from build123d import *

# Parameters (mm, degrees)
SKETCH1_R           = 36
SKETCH1_R_2         = 31.1
BOSS_EXTRUDE1_DEPTH = 15
SKETCH2_R           = 36
BOSS_EXTRUDE2_DEPTH = 5
SKETCH3_R           = 22.5
CUT_EXTRUDE1_DEPTH  = 5
SKETCH4_R           = 5
BOSS_EXTRUDE3_DEPTH = 20
SKETCH7_R           = 2.25
CUT_EXTRUDE2_DEPTH  = 21


with BuildPart() as part:
    # Sketch1 → Boss-Extrude1 (new body)
    with BuildSketch(Plane.XY):
        Circle(SKETCH1_R)
        Circle(SKETCH1_R_2, mode=Mode.SUBTRACT)
    extrude(amount=BOSS_EXTRUDE1_DEPTH)

    # Sketch2 → Boss-Extrude2 (add)
    with BuildSketch(Plane.XY.offset(15)):
        Circle(SKETCH2_R)
    extrude(amount=BOSS_EXTRUDE2_DEPTH)

    # Sketch3 → Cut-Extrude1 (cut)
    with BuildSketch(Plane.XY.offset(20)):
        Circle(SKETCH3_R)
    extrude(amount=-CUT_EXTRUDE1_DEPTH, mode=Mode.SUBTRACT)

    # Sketch4 → Boss-Extrude3 (add)
    with BuildSketch(Plane(origin=(0, 0, 0), x_dir=(-1, 0, 0), z_dir=(0, 0, -1))):
        with Locations((0, 36.1)):
            Circle(SKETCH4_R)
        with Locations((31.263517077, 18.05)):
            Circle(SKETCH4_R)
        with Locations((31.263517077, -18.05)):
            Circle(SKETCH4_R)
        with Locations((0, -36.1)):
            Circle(SKETCH4_R)
        with Locations((-31.263517077, -18.05)):
            Circle(SKETCH4_R)
        with Locations((-31.263517077, 18.05)):
            Circle(SKETCH4_R)
    extrude(amount=-BOSS_EXTRUDE3_DEPTH)

    # Sketch7 → Cut-Extrude2 (cut, through all)
    with BuildSketch(Plane(origin=(0, 0, 0), x_dir=(-1, 0, 0), z_dir=(0, 0, -1))):
        with Locations((-31.263517077, 18.05)):
            Circle(SKETCH7_R)
        with Locations((0, 36.1)):
            Circle(SKETCH7_R)
        with Locations((31.263517077, 18.05)):
            Circle(SKETCH7_R)
        with Locations((31.263517077, -18.05)):
            Circle(SKETCH7_R)
        with Locations((0, -36.1)):
            Circle(SKETCH7_R)
        with Locations((-31.263517077, -18.05)):
            Circle(SKETCH7_R)
    extrude(amount=-CUT_EXTRUDE2_DEPTH, mode=Mode.SUBTRACT)


solid = part.part
Input: part model. Units: mm. Frame: model coordinates. A direction names the side the tool comes from. Give positions to 0.01 mm unless a question says otherwise; leave off trailing zeros. Loops run counter-clockwise (first coordinate to the right, second up) from the corner with the lowest first, then second, coordinate; pieces in that order, holes last. Notation, with made-up numbers: M -12.5,61.5 L 34.5,61.5 A21 ccw 34.5,79.5 Z; hole C 11,-15.5 d9. An arc over 180 degrees is marked long. Use one line per item in the form item = value.
1. Section query A-A, the plane y = 0. Return the cut outline in (x, z), and give its area (3 significant figures).
Numbers:
outline = M -36,0 L -31.1,0 L -31.1,15 L -22.5,15 L -22.5,20 L -36,20 Z; M 22.5,15 L 31.1,15 L 31.1,0 L 36,0 L 36,20 L 22.5,20 Z
area = 282 mm²
2. Section query B-B, the plane z = 9.25. Return the cut outline in (x, y), and give its area (3 significant figures).
Numbers:
outline = M -33.37,-13.51 A5 ccw long -28.39,-22.14 A36 ccw -4.98,-35.65 A5 ccw long 4.98,-35.65 A36 ccw 28.39,-22.14 A5 ccw long 33.37,-13.51 A36 ccw 33.37,13.51 A5 ccw long 28.39,22.14 A36 ccw 4.98,35.65 A5 ccw long -4.98,35.65 A36 ccw -28.39,22.14 A5 ccw long -33.37,13.51 A36 ccw Z; hole C -31.26,-18.05 d4.5; hole C -31.26,18.05 d4.5; hole C 0,0 d62.2; hole C 0,-36.1 d4.5; hole C 0,36.1 d4.5; hole C 31.26,-18.05 d4.5; hole C 31.26,18.05 d4.5
area = 1,190 mm²
3. Section query D-D, the plane y = 18.05. Return the cut outline in (x, z).
Numbers:
outline = M -36.26,0 L -33.51,0 L -33.51,20 L -36.26,20 Z; M -29.01,0 L -25.33,0 L -25.33,15 L -13.43,15 L -13.43,20 L -29.01,20 Z; M 13.43,15 L 25.33,15 L 25.33,0 L 29.01,0 L 29.01,20 L 13.43,20 Z; M 33.51,0 L 36.26,0 L 36.26,20 L 33.51,20 Z
4. Section query C-C, the plane x = 0. Return the cut outline in (y, z).
Numbers:
outline = M -41.1,0 L -38.35,0 L -38.35,20 L -41.1,20 Z; M -33.85,0 L -31.1,0 L -31.1,15 L -22.5,15 L -22.5,20 L -33.85,20 Z; M 22.5,15 L 31.1,15 L 31.1,0 L 33.85,0 L 33.85,20 L 22.5,20 Z; M 38.35,0 L 41.1,0 L 41.1,20 L 38.35,20 Z
5. Reachability of faces 1 (the face through (-6.74, -30.36, 7.4)), 2 (the face through (29.185, -18.912, 9.86)) from +Z, -Z, +X, -X, +Y, -Y: full face, straight path, thin tool, end or side. Return the list, or none.
Numbers:
face_1 = -Z
face_2 = +Z, -Z
6. Line query: L1, parallel to Y at x = 0, z = 16.9; L2, parallel to Y at x = 0, z = 4.75; L3, parallel to Z at x = -20, y = 22. Output: solid intervals per line, ascending.
Numbers:
L1 = -41.1 to -38.35, -33.85 to -22.5, 22.5 to 33.85, 38.35 to 41.1
L2 = -41.1 to -38.35, -33.85 to -31.1, 31.1 to 33.85, 38.35 to 41.1
L3 = 15 to 20
7. First-contact query: pin 1 (7 mm diameter, centred on x = 0, y = -36.1, fed in from +Z); pin 2 (2.5 mm diameter, centred on x = -31.26, y = -18.05, fed in from -Z); pin 3 (3 mm diameter, centred on x = -28, z = 3, fed in from -Y); pin 4 (2 mm diameter, centred on y = -31, z = 5, fed in from -X). Flat tips, straight axial feed; report the tip coordinate or a pass-through.
Numbers:
pin_1 = 20
pin_2 = through
pin_3 = -24.37
pin_4 = -19.9
